Could you check a few things on this model? Use its own coordinates, in mm. A direction names the side the tool comes from. Coordinates: 2 decimals unless noted, no trailing zeros. Loops run counter-clockwise (first coordinate to the right, second up) from the corner with the lowest first, then second, coordinate; pieces in that order, holes last.
from build123d import *

# Parameters (mm, degrees)
SKETCH4_W               = 7.5
SKETCH4_H               = 12
BOSS_EXTRUDE2_DEPTH     = 30
CUT_EXTRUDE1_DEPTH      = 48.571656477
CUT_EXTRUDE1_DEPTH_BACK = 48.571656477
CUT_EXTRUDE2_DEPTH      = 48.571656477
CUT_EXTRUDE2_DEPTH_BACK = 48.571656477
M8_TAPPED_HOLE2_D       = 6.8
M8_TAPPED_HOLE2_DEPTH   = 20
M8_TAPPED_HOLE2_TIP     = 2.042926105
FILLET1_R               = 4
FILLET2_R               = 4


with BuildPart() as part:
    # Sketch2 → Revolve1 (revolve)
    with BuildSketch(Plane(origin=(0, 0, 0), x_dir=(1, 0, 0), z_dir=(0, 1, 0)), mode=Mode.PRIVATE) as revolve1_sk:
        Polygon((-6, 0), (0, 0), (0, 35), (-8, 35), (-8, 27.5), (-8, 15.5), (-8, 12.5), (-6, 12.5), align=None)
    revolve(revolve1_sk.sketch.rotate(Axis((0, 0, 0), (0, 0, -1)), 180), axis=Axis((0, 0, 0), (0, 0, -1)))

    # Sketch4 → Boss-Extrude2 (add, symmetric)
    with BuildSketch(Plane(origin=(0, 0, 0), x_dir=(1, 0, 0), z_dir=(0, 1, 0))):
        with Locations((0, 21.5)):
            Rectangle(SKETCH4_W, SKETCH4_H)
    extrude(amount=BOSS_EXTRUDE2_DEPTH, both=True)

    # Sketch5 → Cut-Extrude1 (cut, two sides: drawn at the far end of the back side and taken through both)
    with BuildSketch(Plane(origin=(3.75, 0, 0), x_dir=(0, 0, -1), z_dir=(1, 0, 0)).offset(-CUT_EXTRUDE1_DEPTH_BACK)):
        Polygon((15.5, 30), (27.5, 23.07179677), (27.5, 30), align=None)
    extrude(amount=CUT_EXTRUDE1_DEPTH + CUT_EXTRUDE1_DEPTH_BACK, mode=Mode.SUBTRACT)

    # Sketch6 → Cut-Extrude2 (cut, two sides: drawn at the far end of the back side and taken through both)
    with BuildSketch(Plane(origin=(3.75, 0, 0), x_dir=(0, 0, -1), z_dir=(1, 0, 0)).offset(-CUT_EXTRUDE2_DEPTH_BACK)):
        Polygon((15.5, -30), (27.5, -23.07179677), (27.5, -30), align=None)
    extrude(amount=CUT_EXTRUDE2_DEPTH + CUT_EXTRUDE2_DEPTH_BACK, mode=Mode.SUBTRACT)

    # M8 Tapped Hole2
    with Locations(Plane.XY):
        with Locations((0, 0)):
            Hole(M8_TAPPED_HOLE2_D / 2, depth=M8_TAPPED_HOLE2_DEPTH)
            with Locations((0, 0, -(M8_TAPPED_HOLE2_DEPTH + M8_TAPPED_HOLE2_TIP / 2))):  # 118° drill point
                Cone(0, M8_TAPPED_HOLE2_D / 2, M8_TAPPED_HOLE2_TIP, mode=Mode.SUBTRACT)

    # Fillet1
    fillet1_edges = [part.edges().sort_by_distance(p)[0] for p in [
        (0, -30, -15.5),
        (0, 30, -15.5),
        (0, 23.07179677, -27.5),
        (0, -23.07179677, -27.5),
    ]]
    fillet(fillet1_edges, radius=FILLET1_R)

    # Fillet2
    # the kernel refuses this fillet: 4 mm, written as the material it takes off along each edge
    with BuildSketch(Plane(origin=(0, 0, -35), x_dir=(1, 0, 0), z_dir=(0, 1, 0))) as fillet2_piece_1:
        with BuildLine():
            CenterArc((8 - FILLET2_R, -FILLET2_R), FILLET2_R, 0, 90)
            Line((8 - FILLET2_R, 0), (8, 0))
            Line((8, 0), (8, -FILLET2_R))
        make_face()
    revolve(axis=Axis((0, 0, -35), (0, 0, -1)), mode=Mode.SUBTRACT)
    with BuildSketch(Plane(origin=(0, 0, -12.5), x_dir=(1, 0, 0), z_dir=(0, 1, 0))) as fillet2_piece_2_section:
        with BuildLine():
            CenterArc((4, 3.464101615), FILLET2_R, 300, 60)
            Line((6, 0), (8, 0))
            Line((8, 0), (8, 3.464101615))
        make_face()
    fillet2_piece_2 = revolve(axis=Axis((0, 0, -12.5), (0, 0, -1)), mode=Mode.PRIVATE)
    fillet2_piece_2 = split(fillet2_piece_2, bisect_by=Plane(origin=(3.75, -4.120033491, -15.73161152), z_dir=(1, 0, 0)), keep=Keep.TOP, mode=Mode.PRIVATE)
    add(fillet2_piece_2, mode=Mode.SUBTRACT)
    with BuildSketch(Plane(origin=(0, 0, -12.5), x_dir=(1, 0, 0), z_dir=(0, 1, 0))) as fillet2_piece_3_section:
        with BuildLine():
            CenterArc((4, 3.464101615), FILLET2_R, 300, 60)
            Line((6, 0), (8, 0))
            Line((8, 0), (8, 3.464101615))
        make_face()
    fillet2_piece_3 = revolve(axis=Axis((0, 0, -12.5), (0, 0, -1)), mode=Mode.PRIVATE)
    fillet2_piece_3 = split(fillet2_piece_3, bisect_by=Plane(origin=(0, -7.348709995, -15.5), z_dir=(0, 0, 1)), keep=Keep.TOP, mode=Mode.PRIVATE)
    add(fillet2_piece_3, mode=Mode.SUBTRACT)
    with BuildSketch(Plane(origin=(0, 0, -12.5), x_dir=(1, 0, 0), z_dir=(0, 1, 0))) as fillet2_piece_4_section:
        with BuildLine():
            CenterArc((4, 3.464101615), FILLET2_R, 300, 60)
            Line((6, 0), (8, 0))
            Line((8, 0), (8, 3.464101615))
        make_face()
    fillet2_piece_4 = revolve(axis=Axis((0, 0, -12.5), (0, 0, -1)), mode=Mode.PRIVATE)
    fillet2_piece_4 = split(fillet2_piece_4, bisect_by=Plane(origin=(-3.75, 0, -15.73161152), z_dir=(-1, 0, 0)), keep=Keep.TOP, mode=Mode.PRIVATE)
    add(fillet2_piece_4, mode=Mode.SUBTRACT)


solid = part.part
1) If I drill on L1, parallel to X at y = -15, z = -23.5; L2, parallel to Y at x = 0, z = -11.5, over which ranges is the centre line in solid material (lowest first)?
2) For faces 4 (the flat face through (-3.75, 17, -21)), 5 (the flat face through (-3.75, -17, -21)), 6 (the flat face through (3.75, 17, -22)), which set-ups out of +Z, -Z, +X, -X, +Y, -Y let a thin tool reach every point of the face, with its end or its side?
3) Imagine slicing it at B-B on y = 17. List the corners of the cut face in (x, z) for me, plus the area to 3 significant figures.
4) Imagine slicing it at C-C on z = -9. List the corners of the cut face in (x, y) for me.
5) Will these pins go through, and if not, where does the flat tip stop? pin 1 (6 mm diameter, centred on y = 18.5, z = -21.5, fed in from -X); pin 2 (4 mm diameter, centred on x = -1, y = 14.5, fed in from +Z); pin 3 (2.5 mm diameter, centred on x = 0.5, y = -11, fed in from -Z); pin 4 (8 mm diameter, centred on x = -2, z = -17, fed in from -Y).
6) We'd pull the mould along X, two halves only. Please class faces 1 (the flat face through (3.75, -17, -21)), 2 (the cylindrical face through (0.053, 26.506, -17.449)), 3 (the cylindrical face through (0.74, -3.32, -10.14)): released by +X, released by -X, zero draft, split by the parting line, or undercut.
7) Imagine slicing it at A-A on z = -17.5. List the corners of the cut face in (x, y) for me, plus the area to 3 significant figures.
Solved:
1. L1: x = -3.75 to 3.75
1. L2: y = -6 to -3.4, 3.4 to 6
2. face 4: +Z, -Z, -X, +Y
2. face 5: +Z, -Z, -X, -Y
2. face 6: +Z, -Z, +X, +Y
3. outline: (-3.75, -27.5) - (3.75, -27.5) - (3.75, -15.5) - (-3.75, -15.5) - close
3. area: 90.0 mm2
4. outline: circle Ø12 at (0, 0); hole circle Ø6.8 at (0, 0)
5. pin 1: stops at x = -3.75
5. pin 2: stops at z = -15.5
5. pin 3: stops at z = -27.5
5. pin 4: stops at y = -27.07
6. face 1: released by +X
6. face 2: zero draft
6. face 3: undercut
7. outline: (-3.75, -26.54) - (3.75, -26.54) - (3.75, -7.07) arc R8 ccw to (3.75, 7.07) - (3.75, 26.54) - (-3.75, 26.54) - (-3.75, 7.07) arc R8 ccw to (-3.75, -7.07) - close; hole circle Ø6.8 at (0, 0)
7. area: 447 mm2
